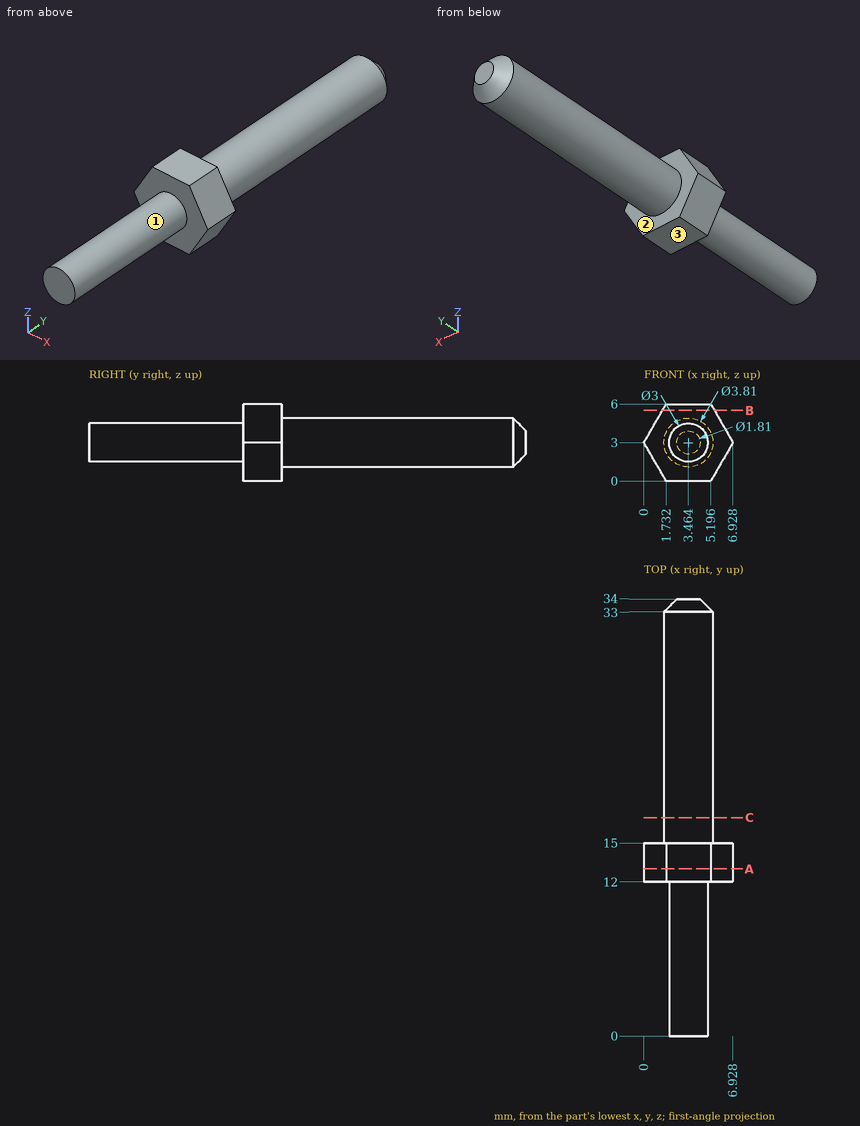
Answer from the drawing. Dimensions are ordinates in mm from the lowest x, y and z of the part. A direction names the side the tool comes from. Give positions to 0.01 mm unless a question says otherwise; leave off trailing zeros. Order: outer loops, then holes, each group sorted by start corner. A loop starts at its lowest first (then second) coordinate and runs counter-clockwise, first axis right, second up. Notation, with made-up numbers: (-3, -17) - (10, -17) arc R22 cw to (10, -3) - close; hole circle Ø8 at (22.25, 10.5). An arc over 180 degrees is marked (long way). One line per item, written item: value. Start each with the question number.
1. Section B-B, the plane z = 5.5 is taken. Write down the section's boundary in (x, y) (1 decimal), then the cut area to 3 significant figures.
2. Each of these flat-tipped pins is pushed along its axis until it touches: pin 1 Ø3 at (x, z) = (3.5, 1.5) entering from -Y; pin 2 Ø1.5 at (y, z) = (3.5, 3) entering from +X; pin 3 Ø4 at (x, y) = (4, 6) entering from +Z; pin 4 Ø2 at (x, z) = (5.5, 5) entering from -Y. Where does it stop, or does it pass through?
3. Section A-A, the plane y = 13 is taken. Write down the section's boundary in (x, z).
4. Which of the six approach directions +Z, -Z, +X, -X, +Y, -Y give full straight-line access (tool end or side, diameter ignored) to the marked faces 1, 2 and 3?
5. Consider line 1 (Z direction, x = 3.5, y = 4); line 2 (Y direction, x = 5.5, z = 2); line 3 (Z direction, x = 5, y = 18). Determine where each line is inside the solid, lowest interval first.
6. Section C-C, the plane y = 17 is taken. Write down the section's boundary in (x, z) (1 decimal), then the cut area to 3 significant figures.
Filled sheet:
1. outline: (1.4, 12) - (5.5, 12) - (5.5, 15) - (1.4, 15) - close
1. area: 12.1 mm²
2. pin 1: y = 0
2. pin 2: x = 4.96
2. pin 3: z = 4.5
2. pin 4: y = 12
3. outline: (0, 3) - (1.73, 0) - (5.2, 0) - (6.93, 3) - (5.2, 6) - (1.73, 6) - close
4. face 1: -Y
4. face 2: +Y
4. face 3: -Z, +X, -X, +Y, -Y
5. line 1: 1.5 to 4.5
5. line 2: 12 to 15
5. line 3: 1.87 to 4.13
6. outline: circle Ø3.8 at (3.5, 3)
6. area: 11.4 mm²
